from build123d import *

# Parameters (mm, degrees)
SKETCH1_R           = 1.58242
BOSS_EXTRUDE1_DEPTH = 113.50625
SKETCH2_R           = 0.79375
CUT_EXTRUDE1_DEPTH  = 3.175
SKETCH3_R           = 0.396875
CUT_EXTRUDE2_DEPTH  = 14.2875
CUT_EXTRUDE4_START  = -14.2875
SKETCH4_R           = 0.79375
CUT_EXTRUDE4_DEPTH  = 100.21875


with BuildPart() as part:
    # Sketch1 → Boss-Extrude1 (new body)
    with BuildSketch(Plane.XY):
        Circle(SKETCH1_R)
    extrude(amount=-BOSS_EXTRUDE1_DEPTH)

    # Sketch2 → Cut-Extrude1 (cut)
    with BuildSketch(Plane.XY):
        Circle(SKETCH2_R)
    extrude(amount=-CUT_EXTRUDE1_DEPTH, mode=Mode.SUBTRACT)

    # Sketch3 → Cut-Extrude2 (cut)
    with BuildSketch(Plane.XY):
        Circle(SKETCH3_R)
    extrude(amount=-CUT_EXTRUDE2_DEPTH, mode=Mode.SUBTRACT)

    # Sketch4 → Cut-Extrude4 (cut, through all)
    with BuildSketch(Plane.XY.offset(CUT_EXTRUDE4_START)):
        Circle(SKETCH4_R)
    extrude(amount=-CUT_EXTRUDE4_DEPTH, mode=Mode.SUBTRACT)

    # Sketch5 → Revolve1 (revolve)
    with BuildSketch(Plane(origin=(0, 0, 0), x_dir=(0, 0, -1), z_dir=(1, 0, 0))):
        with BuildLine():
            Line((12.7, 1.58242), (13.752029901, 2.111801446))
            ThreePointArc((13.752029901, 2.111801446), (14.2875, 2.238931679), (14.822970099, 2.111801446))
            Line((14.822970099, 2.111801446), (15.875, 1.58242))
            Line((15.875, 1.58242), (12.7, 1.58242))
        make_face()
    revolve(axis=Axis((0, 0, 0), (0, 0, -1)))


solid = part.part
Check sheet for the modelled part. Datum: model origin and axes. Units: mm. A direction names the side the tool comes from. Give positions to 0.01 mm unless a question says otherwise; leave off trailing zeros. Order: outer loops, then holes, each group sorted by start corner. A loop starts at its lowest first (then second) coordinate and runs counter-clockwise, first axis right, second up. Notation, with made-up numbers: (2.5, -3.75) - (57.5, -3.75) arc R18 cw to (57.5, 27.25) - close; hole circle Ø3 at (10, 51). An arc over 180 degrees is marked (long way). Answer as CSV lines item,"result".
1. Tool access check on faces 1 (the face through (1.46, -0.61, -6.26)), 2 (the face through (-1, 0, 0)), 3 (the face through (1.46, -0.61, -64.01)). Record the directions out of +Z, -Z, +X, -X, +Y, -Y that give a thin tool (end or side, any length) a straight path to the whole face; none if there is none.
Result sheet:
face 1,"+Z"
face 2,"+Z, +X, -X, +Y, -Y"
face 3,"-Z"
2. Scan lines: probe 1 along Y at (x, z) = (0, -42.5); probe 2 along Y at (x, z) = (0, -6). Record each from-to range of solid material in increasing order. Write a range as from..to.
Result sheet:
probe 1,"-1.58..-0.79, 0.79..1.58"
probe 2,"-1.58..-0.4, 0.4..1.58"
3. Section check A-A (z = -40). Record the boundary of the cut face in (x, y).
Result sheet:
outline,"circle Ø3.16 at (0, 0); hole circle Ø1.59 at (0, 0)"
4. Go/stop test with flat-tipped pins: P1, Ø1, axis at y = 0, z = -73.5, coming from the -X side; P2, Ø1, axis at x = 0, y = 0, coming from the -Z side; P3, Ø1.3, axis at x = 0, y = 0, coming from the +Z side (3 decimals). Record where each tip stops, or that it passes through.
Result sheet:
P1,"x = -1.58"
P2,"z = -14.29"
P3,"z = -3.175"
